Geometry: final body of the model. Coordinates: model frame, mm. Face numbers are marked on the shaded views. Give positions to 0.01 mm unless a question says otherwise; leave off trailing zeros. Loops run counter-clockwise (first coordinate to the right, second up) from the corner with the lowest first, then second, coordinate; pieces in that order, holes last.
1. First-contact query: P1, Ø6, axis at x = 187, y = 20, coming from the -Z side; P2, Ø9, axis at y = -3.5, z = 285, coming from the +X side; P3, Ø3, axis at y = -19, z = -187, coming from the +X side. Flat tips, straight axial feed; report the tip coordinate or a pass-through.
2. Section B-B, the plane x = 0. Output: boundary loops of the cut face in (y, z), then the cut area to 3 significant figures.
3. Section A-A, the plane z = 0. Output: boundary loops of the cut face in (x, y), then the cut area to 3 significant figures.
4. Section D-D, the plane z = 182. Output: boundary loops of the cut face in (x, y), then the cut area to 3 significant figures.
5. Material intervals for line 1 along X through (y, z) = (-8.5, -239.5); line 2 along Z through (x, y) = (270.5, 10); line 3 along Y through (x, z) = (29.5, -293.5), sorted ascending.
6. Draft query along X for the marked faces 1, 2 and 3. Return one class per face: +X half, -X half, draft (parallel to the pull), parting line (faces both ways), or undercut.
7. Section C-C, the plane y = -6. State how many separate pieces and enclosed holes the cut face has, then the cut area to 3 significant figures.
from build123d import *

# Parameters (mm, degrees)
SKETCH1_R           = 320
SKETCH1_R_2         = 270
BOSS_EXTRUDE1_DEPTH = 30
SKETCH2_W           = 60
SKETCH2_H           = 30
CUT_EXTRUDE1_DEPTH  = 454.541618818
CIRPATTERN1_COUNT   = 10
SKETCH3_R           = 5
CUT_EXTRUDE2_DEPTH  = 457.508488421
CIRPATTERN2_COUNT   = 10


with BuildPart() as part:
    # Sketch1 → Boss-Extrude1 (new, symmetric)
    with BuildSketch(Plane(origin=(0, 0, 0), x_dir=(1, 0, 0), z_dir=(0, 1, 0))):
        with Locations(Location((0, 0, 0), (0, 0, 270))):
            Circle(SKETCH1_R)
        with Locations(Location((0, 0, 0), (0, 0, 270))):
            Circle(SKETCH1_R_2, mode=Mode.SUBTRACT)
    extrude(amount=BOSS_EXTRUDE1_DEPTH, both=True)

    # Sketch2 → Cut-Extrude1 (cut, symmetric)
    with BuildSketch(Plane.XY):
        Rectangle(SKETCH2_W, SKETCH2_H)
    cut_extrude1 = extrude(amount=CUT_EXTRUDE1_DEPTH, both=True, mode=Mode.SUBTRACT)

    # CirPattern1: Cut-Extrude1 ×10 about axis
    cirpattern1_axis = Axis((0, 0, 0), (0, 1, 0))
    for i in range(1, CIRPATTERN1_COUNT):
        add(cut_extrude1.rotate(cirpattern1_axis, i * 360 / CIRPATTERN1_COUNT), mode=Mode.SUBTRACT)

    # Sketch3 → Cut-Extrude2 (cut, through all)
    with BuildSketch(Plane(origin=(0, 30, 0), x_dir=(1, 0, 0), z_dir=(0, 1, 0))):
        with Locations(Location((-15, 303, 0), (0, 0, 270))):
            Circle(SKETCH3_R)
        with Locations(Location((15, 303, 0), (0, 0, 270))):
            Circle(SKETCH3_R)
    cut_extrude2 = extrude(amount=-CUT_EXTRUDE2_DEPTH, mode=Mode.SUBTRACT)

    # CirPattern2: Cut-Extrude2 ×10 about axis
    cirpattern2_axis = Axis((0, 0, 0), (0, 1, 0))
    for i in range(1, CIRPATTERN2_COUNT):
        add(cut_extrude2.rotate(cirpattern2_axis, i * 360 / CIRPATTERN2_COUNT), mode=Mode.SUBTRACT)


solid = part.part
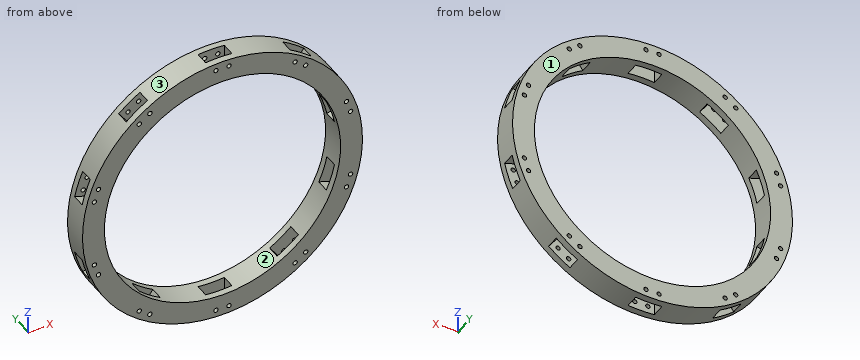
Answers below:
1. P1: stops at z = -261.81
1. P2: stops at x = 154.01
1. P3: stops at x = 260.75
2. outline: (-30, -320) - (-15, -320) - (-15, -270) - (-30, -270) - close; (-30, 270) - (-15, 270) - (-15, 320) - (-30, 320) - close; (15, -320) - (30, -320) - (30, -270) - (15, -270) - close; (15, 270) - (30, 270) - (30, 320) - (15, 320) - close
2. area: 3,000 mm2
3. outline: (-320, -30) - (-270, -30) - (-270, 30) - (-320, 30) - close; (270, -30) - (320, -30) - (320, 30) - (270, 30) - close
3. area: 6,000 mm2
4. outline: (-263.2, -30) - (-199.44, -30) - (-199.44, 30) - (-263.2, 30) - close; (199.44, -30) - (263.2, -30) - (263.2, 30) - (199.44, 30) - close
4. area: 7,650 mm2
5. line 1: x = -212.23 to -211.09, -136.92 to -124.66, 124.66 to 136.92, 211.09 to 212.23
5. line 2: z = -170.97 to -119.43, -56.35 to 56.35, 119.43 to 170.97
5. line 3: y = -30 to -15, 15 to 30
6. face 1: draft
6. face 2: undercut
6. face 3: parting line
7. separate pieces: 10
7. enclosed holes: 0
7. area: 62,600 mm2
